```python
from build123d import *

# Parameters (mm, degrees)
F0_W       = 3
F0_H       = 10
F1_DEPTH   = 20
F2_D       = 6
F5_D       = 8
F5_ON_F4_D = 8


with BuildPart() as f1:
    # F0 (on Top) → F1 (new body)
    with BuildSketch(Plane.XY):
        with BuildLine():
            ThreePointArc((-12.3592070943, 8.5), (-14.3245960923, 4.4503872632), (-15, 0))
            Line((-15, 0), (-9.5, 0))
            ThreePointArc((-9.5, 0), (-8.0794519161, 4.9972449146), (-4.2426406871, 8.5))
            Line((-4.2426406871, 8.5), (-12.3592070943, 8.5))
        make_face()
        with BuildLine():
            Line((4.2426406871, 8.5), (12.3592070943, 8.5))
            ThreePointArc((12.3592070943, 8.5), (0.1020002099, 14.9996531946), (-12.2424665449, 8.667295593))
            ThreePointArc((-12.2424665449, 8.667295593), (-12.301121226, 8.5838462581), (-12.3592070943, 8.5))
            Line((-12.3592070943, 8.5), (-4.2426406871, 8.5))
            ThreePointArc((-4.2426406871, 8.5), (0, 9.5), (4.2426406871, 8.5))
        make_face()
        with BuildLine():
            Line((-9.5, 0), (9.5, 0))
            ThreePointArc((9.5, 0), (8.0794519161, 4.9972449146), (4.2426406871, 8.5))
            Line((4.2426406871, 8.5), (-4.2426406871, 8.5))
            ThreePointArc((-4.2426406871, 8.5), (-8.0794519161, 4.9972449146), (-9.5, 0))
        make_face()
        with BuildLine():
            Line((-4.2426406871, 8.5), (4.2426406871, 8.5))
            ThreePointArc((4.2426406871, 8.5), (0, 9.5), (-4.2426406871, 8.5))
        make_face()
        with BuildLine():
            Line((9.5, 0), (15, 0))
            ThreePointArc((15, 0), (14.3245960923, 4.4503872632), (12.3592070943, 8.5))
            Line((12.3592070943, 8.5), (4.2426406871, 8.5))
            ThreePointArc((4.2426406871, 8.5), (8.0794519161, 4.9972449146), (9.5, 0))
        make_face()
        with BuildLine():
            ThreePointArc((-9.5, 0), (0, -9.5), (9.5, 0))
            Line((9.5, 0), (-9.5, 0))
        make_face()
        with BuildLine():
            Line((-11, -19.2), (11, -19.2))
            Line((11, -19.2), (11, -9.2))
            Line((11, -9.2), (15, -9.2))
            Line((15, -9.2), (15, 0))
            Line((15, 0), (9.5, 0))
            ThreePointArc((9.5, 0), (0, -9.5), (-9.5, 0))
            Line((-9.5, 0), (-15, 0))
            Line((-15, 0), (-15, -9.2))
            Line((-15, -9.2), (-11, -9.2))
            Line((-11, -9.2), (-11, -19.2))
        make_face()
        Polygon((-28, -19.2), (-11, -19.2), (-11, -9.2), (-15, -9.2), (-28, -9.2), align=None)
        with Locations((-29.5, -14.2)):
            Rectangle(F0_W, F0_H)
        Polygon((11, -19.2), (28, -19.2), (28, -9.2), (15, -9.2), (11, -9.2), align=None)
        with Locations((29.5, -14.2)):
            Rectangle(F0_W, F0_H)
    extrude(amount=-F1_DEPTH)

    # F2 (through all)
    with Locations(Plane.XY):
        with Locations((0, 0)):
            Hole(F2_D / 2)

    # F5 (through all)
    with Locations(Plane(origin=(0, -9.2, 0), x_dir=(-1, 0, 0), z_dir=(0, 1, 0))):
        with Locations((-23, -10)):
            Hole(F5_D / 2)

    # F5 on F4 (through all)
    with Locations(Plane(origin=(0, -9.2, 0), x_dir=(-1, 0, 0), z_dir=(0, 1, 0))):
        with Locations((23, -10)):
            Hole(F5_ON_F4_D / 2)


solid = f1.part
```
Build history of the part. All positions in model axes, mm. A direction names the side the tool comes from. Round coordinates to 2 decimals unless told otherwise and drop trailing zeros. Write each loop counter-clockwise with the first axis right and the second up, starting at its lowest first coordinate (ties: lowest second). Pieces come first, ordered by that corner, then holes. Notation, with made-up numbers: (53, 74.5) - (105, 74.5) arc R28 ccw to (105, 108.5) - close; hole circle Ø5 at (-20, 11.5). An arc over 180 degrees is marked (long way). Answer as CSV lines item,"result".
Q1. Pull direction Z, two halves, no side cores. Call faces 4 (the flat face through (31, -14, -10)), 5 (the cylindrical face through (-26.2, -14.3, -12.4)), 6 (the flat face through (0, -6, 0)): +Z half, -Z half, draft (parallel to the pull), parting line (faces both ways), or undercut.
Report:
face 4,"draft"
face 5,"undercut"
face 6,"+Z half"
Q2. Drill centre lines: probe 1 along Y at (x, z) = (0, -13.75); probe 2 along Y at (x, z) = (-21.5, -3.5); probe 3 along X at (y, z) = (-12.5, -6.5). Where is each one in solid material? Low to high. Write a range as [from, to].
Report:
probe 1,"y = [-19.2, -3], [3, 15]"
probe 2,"y = [-19.2, -9.2]"
probe 3,"x = [-31, -24.94], [-21.06, 21.06], [24.94, 31]"
Q3. Cut at C-C (z = -4.25). Write the cut outline in (x, y).
Report:
outline,"(-31, -19.2) - (31, -19.2) - (31, -9.2) - (15, -9.2) - (15, 0) arc R15 ccw to (-15, 0) - (-15, -9.2) - (-31, -9.2) - close; hole circle Ø6 at (0, 0)"
Q4. Cut at A-A (z = -10). Write the cut outline in (x, y).
Report:
outline,"(-31, -19.2) - (-27, -19.2) - (-27, -9.2) - (-31, -9.2) - close; (-19, -19.2) - (19, -19.2) - (19, -9.2) - (15, -9.2) - (15, 0) arc R15 ccw to (-15, 0) - (-15, -9.2) - (-19, -9.2) - close; (27, -19.2) - (31, -19.2) - (31, -9.2) - (27, -9.2) - close; hole circle Ø6 at (0, 0)"
Q5. Drop flat-ended pins along their axis: pin 1 (8 mm diameter, centred on x = 2.5, y = 8.5, fed in from +Z); pin 2 (12 mm diameter, centred on x = 18.5, z = -13.5, fed in from +Y); pin 3 (3 mm diameter, centred on y = -3, z = -12, fed in from -X); pin 4 (5 mm diameter, centred on x = -23, z = -10, fed in from +Y). Give the stop position or say it passes through.
Report:
pin 1,"stops at z = 0"
pin 2,"stops at y = 8.29"
pin 3,"stops at x = -15"
pin 4,"passes through"
Q6. Cut at B-B (x = 23). Write the cut outline in (y, z).
Report:
outline,"(-19.2, -20) - (-9.2, -20) - (-9.2, -14) - (-19.2, -14) - close; (-19.2, -6) - (-9.2, -6) - (-9.2, 0) - (-19.2, 0) - close"
Q7. Cut at D-D (y = -1.5). Write the cut outline in (x, z), and give its area (3 significant figures).
Report:
outline,"(-15, -20) - (-2.6, -20) - (-2.6, 0) - (-15, 0) - close; (2.6, -20) - (15, -20) - (15, 0) - (2.6, 0) - close"
area,"496 mm^2"
Q8. Tool access for faces 1 (the cylindrical face through (3, 0, -10)), 2 (the flat face through (-19, -9.2, -8)), 3 (the flat face through (15, -5, -10)): list every direction of +Z, -Z, +X, -X, +Y, -Y with a clear straight run to the whole face (end or side of a thin tool).
Report:
face 1,"+Z, -Z"
face 2,"+Z, -Z, -X, +Y"
face 3,"+Z, -Z, +X, +Y"
